Input: part model. Units: mm. Frame: model coordinates. Coordinates: 2 decimals unless noted, no trailing zeros. Write each loop counter-clockwise with the first axis right and the second up, starting at its lowest first coordinate (ties: lowest second). Pieces come first, ordered by that corner, then holes. Notation, with made-up numbers: M 54,26.25 L 70,26.25 A21 ccw 70,61.25 Z; hole C -4.75,-5.75 d6. An arc over 180 degrees is marked long. Write each question's results on one line, items separated by ' | '. Start each with the question number.
1. Section query B-B, the plane y = 2.05. Output: boundary loops of the cut face in (x, z).
2. Section query C-C, the plane x = 0. Output: boundary loops of the cut face in (y, z) (3 decimals), and give its area (3 significant figures).
3. Ray query, probe 1 along Z at (x, y) = (-25.4, 1); probe 2 along Z at (x, y) = (11, 2.5). Return the intervals inside material, ascending.
4. Section query A-A, the plane z = 0. Output: boundary loops of the cut face in (x, y) (3 decimals).
5. Section query D-D, the plane x = 25.5. Output: boundary loops of the cut face in (y, z) (3 decimals), and give its area (3 significant figures).
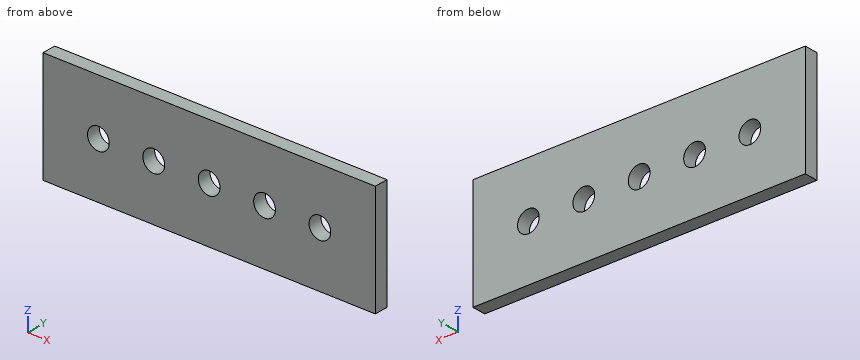
Autodesk Inventor part; units mm, degrees
ref_plane "YZ Plane" through (0, 0, 0) normal (1, 0, 0) x (0, 1, 0)
ref_plane "XZ Plane" through (0, 0, 0) normal (0, 1, 0) x (-1, 0, 0)
ref_plane "XY Plane" through (0, 0, 0) normal (0, 0, 1) x (1, 0, 0)
sketch "Sketch1" plane through (0, 0, 0) normal (0, 1, 0) x (-1, 0, 0)
  line L0 (38.1, 12.7) -> (-38.1, 12.7)
  line L1 (-38.1, 12.7) -> (-38.1, -12.7)
  line L2 (-38.1, -12.7) -> (38.1, -12.7)
  line L3 (38.1, -12.7) -> (38.1, 12.7)
  line L4 (38.1, 12.7) -> (-38.1, -12.7) construction
  line L5 (-38.1, 12.7) -> (38.1, -12.7) construction
  circle A0 centre (25.4, 0) radius 2.4892
  circle A1 centre (12.7, 0) radius 2.4892
  circle A2 centre (0, 0) radius 2.4892
  circle A3 centre (-12.7, 0) radius 2.4892
  circle A4 centre (-25.4, 0) radius 2.4892
  point P0 (0, 0)
  point P1 (38.1, 0)
  dimension "d0" = 76.2
  dimension "d1" = 25.4
  dimension "d2" = 4.9784
  dimension "d3" = 12.7
  dimension "d4" = 12.7
  dimension "d7" = 12.7
  dimension "d12" = 12.7
  dimension "d13" = 12.7
extrude "Extrusion1" add sketch "Sketch1" along normal blind 3.175
properties part number "1x5-Grid-Gusset"
Answer:
1) outline: M -38.1,-12.7 L 38.1,-12.7 L 38.1,12.7 L -38.1,12.7 Z; hole C -25.4,0 d4.98; hole C -12.7,0 d4.98; hole C 0,0 d4.98; hole C 12.7,0 d4.98; hole C 25.4,0 d4.98
2) outline: M 0,-12.7 L 3.175,-12.7 L 3.175,-2.489 L 0,-2.489 Z; M 0,2.489 L 3.175,2.489 L 3.175,12.7 L 0,12.7 Z | area: 64.8 mm^2
3) probe 1: -12.7 to -2.49, 2.49 to 12.7 | probe 2: -12.7 to -1.82, 1.82 to 12.7
4) outline: M -38.1,0 L -27.889,0 L -27.889,3.175 L -38.1,3.175 Z; M -22.911,0 L -15.189,0 L -15.189,3.175 L -22.911,3.175 Z; M -10.211,0 L -2.489,0 L -2.489,3.175 L -10.211,3.175 Z; M 2.489,0 L 10.211,0 L 10.211,3.175 L 2.489,3.175 Z; M 15.189,0 L 22.911,0 L 22.911,3.175 L 15.189,3.175 Z; M 27.889,0 L 38.1,0 L 38.1,3.175 L 27.889,3.175 Z
5) outline: M 0,-12.7 L 3.175,-12.7 L 3.175,-2.487 L 0,-2.487 Z; M 0,2.487 L 3.175,2.487 L 3.175,12.7 L 0,12.7 Z | area: 64.9 mm^2
